Part model, mm, in its own coordinate system. A direction names the side the tool comes from. Round coordinates to 2 decimals unless told otherwise and drop trailing zeros. Loops run counter-clockwise (first coordinate to the right, second up) from the corner with the lowest first, then second, coordinate; pieces in that order, holes last. Notation, with made-up numbers: (-26, 82.5) - (15, 82.5) arc R27 cw to (15, 102.5) - close; hole circle Ø11 at (79.25, 16). An arc over 180 degrees is marked (long way). Write each question's results on one line, items separated by ' | '. Start each with the question number.
(1) Flat gauge pin, fed straight in: P1, Ø3.5, axis at x = 25.25, y = 20, coming from the -Z side. Where does the tip first touch, or does it go through?
(2) Cut at C-C, the plane x = 53.5. List the corners of the cut face in (y, z).
(3) Cut at D-D, the plane z = 1. Give the number of separate pieces and of enclosed holes in the cut face, then the cut area to 3 significant figures.
(4) Cut at A-A, the plane x = 6. List the corners of the cut face in (y, z).
(5) Mould opens along X. For faces 3 (the face through (10.6, -19.14, 0.99)), 4 (the face through (-12, 0, 0)), 5 (the face through (-76.64, 24.1, 1.01)) say: released by +X, released by -X, zero draft, split by the parting line, or undercut.
(6) Cut at B-B, the plane y = -8. List the corners of the cut face in (x, z).
(7) Tool access for faces 1 (the face through (29.15, 22.14, 0.99)), 2 (the face through (-76.64, -24.1, 1.01)): list every direction of +Z, -Z, +X, -X, +Y, -Y with a clear straight run to the whole face (end or side of a thin tool).
(8) Drill centre lines: L1, parallel to X at y = 10.5, z = 1.7; L2, parallel to X at y = 4.5, z = 1; L3, parallel to Y at x = -74.25, z = 1.4. Where is each one in solid material? Low to high.
from build123d import *

# Parameters (mm, degrees)
SKETCH_1_W          = 155
SKETCH_1_H          = 50
EXTRUDE_1_DEPTH     = 2
SKETCH_2_R          = 1.5
CUT_EXTRUDE_1_DEPTH = 10
FILLET_1_R          = 3
SKETCH_3_W          = 43
SKETCH_3_H          = 46
CUT_EXTRUDE_2_DEPTH = 10
FILLET_2_R          = 3
SKETCH_4_W          = 23
SKETCH_4_H          = 40
CUT_EXTRUDE_3_DEPTH = 10
FILLET_3_R          = 3
SKETCH_5_R          = 4.732430395
SKETCH_5_R_2        = 4.815282463
SKETCH_5_R_3        = 4.035251629
CUT_EXTRUDE_4_DEPTH = 10


with BuildPart() as part:
    # 草图1 → 凸台-拉伸1 (new body)
    with BuildSketch(Plane.XY):
        Rectangle(SKETCH_1_W, SKETCH_1_H)
    extrude(amount=EXTRUDE_1_DEPTH)

    # 草图2 → 切除-拉伸1 (cut)
    with BuildSketch(Plane(origin=(0, 0, 0), x_dir=(-1, 0, 0), z_dir=(0, 0, -1))):
        with Locations((-25.25, -20)):
            Circle(SKETCH_2_R)
        with Locations((-74.25, -20)):
            Circle(SKETCH_2_R)
        with Locations((-25.25, 20)):
            Circle(SKETCH_2_R)
        with Locations((-74.25, 20)):
            Circle(SKETCH_2_R)
        with Locations((25.25, -20)):
            Circle(SKETCH_2_R)
        with Locations((74.25, -20)):
            Circle(SKETCH_2_R)
        with Locations((25.25, 20)):
            Circle(SKETCH_2_R)
        with Locations((74.25, 20)):
            Circle(SKETCH_2_R)
        with Locations((16, 2.5)):
            Circle(SKETCH_2_R)
        with Locations((16, 17.5)):
            Circle(SKETCH_2_R)
        with Locations((-16, 2.5)):
            Circle(SKETCH_2_R)
        with Locations((-16, 17.5)):
            Circle(SKETCH_2_R)
    extrude(amount=-CUT_EXTRUDE_1_DEPTH, mode=Mode.SUBTRACT)

    # 圆角1
    fillet_1_edges = [part.edges().sort_by_distance(p)[0] for p in [
        (77.5, -25, 1),
        (-77.5, -25, 1),
        (-77.5, 25, 1),
        (77.5, 25, 1),
    ]]
    fillet(fillet_1_edges, radius=FILLET_1_R)

    # 草图3 → 切除-拉伸2 (cut)
    with BuildSketch(Plane.XY.offset(2)):
        with Locations((49.75, 0)):
            Rectangle(SKETCH_3_W, SKETCH_3_H)
        with Locations((-49.75, 0)):
            Rectangle(SKETCH_3_W, SKETCH_3_H)
    extrude(amount=-CUT_EXTRUDE_2_DEPTH, mode=Mode.SUBTRACT)

    # 圆角2
    fillet_2_edges = [part.edges().sort_by_distance(p)[0] for p in [
        (71.25, 23, 1),
        (71.25, -23, 1),
        (28.25, -23, 1),
        (28.25, 23, 1),
        (-28.25, 23, 1),
        (-28.25, -23, 1),
        (-71.25, -23, 1),
        (-71.25, 23, 1),
    ]]
    fillet(fillet_2_edges, radius=FILLET_2_R)

    # 草图4 → 切除-拉伸3 (cut)
    with BuildSketch(Plane.XY.offset(2)):
        Rectangle(SKETCH_4_W, SKETCH_4_H)
    extrude(amount=-CUT_EXTRUDE_3_DEPTH, mode=Mode.SUBTRACT)

    # 圆角3
    fillet_3_edges = [part.edges().sort_by_distance(p)[0] for p in [
        (11.5, 20, 1),
        (11.5, -20, 1),
        (-11.5, -20, 1),
        (-11.5, 20, 1),
    ]]
    fillet(fillet_3_edges, radius=FILLET_3_R)

    # 草图5 → 切除-拉伸4 (cut)
    with BuildSketch(Plane.XY.offset(2)):
        with Locations((19.907240007, 10.387913302)):
            Circle(SKETCH_5_R)
        with Locations((18.386877163, -5.018430181)):
            Circle(SKETCH_5_R_2)
        with Locations((16.663799274, -17.890835592)):
            Circle(SKETCH_5_R_3)
        with Locations(Location((-16.663799274, -17.890835592, 0), (0, 0, 180))):
            Circle(SKETCH_5_R_3)
        with Locations(Location((-18.386877163, -5.018430181, 0), (0, 0, 180))):
            Circle(SKETCH_5_R_2)
        with Locations(Location((-19.907240007, 10.387913302, 0), (0, 0, 180))):
            Circle(SKETCH_5_R)
    extrude(amount=-CUT_EXTRUDE_4_DEPTH, mode=Mode.SUBTRACT)


solid = part.part
A:
1) P1: z = 0
2) outline: (-25, 0) - (-23, 0) - (-23, 2) - (-25, 2) - close; (23, 0) - (25, 0) - (25, 2) - (23, 2) - close
3) separate pieces: 1 | enclosed holes: 21 | area: 2,420 mm2
4) outline: (-25, 0) - (-20, 0) - (-20, 2) - (-25, 2) - close; (20, 0) - (25, 0) - (25, 2) - (20, 2) - close
5) face 3: undercut | face 4: zero draft | face 5: released by -X
6) outline: (-77.5, 0) - (-71.25, 0) - (-71.25, 2) - (-77.5, 2) - close; (-28.25, 0) - (-22.17, 0) - (-22.17, 2) - (-28.25, 2) - close; (-14.61, 0) - (-11.5, 0) - (-11.5, 2) - (-14.61, 2) - close; (11.5, 0) - (14.61, 0) - (14.61, 2) - (11.5, 2) - close; (22.17, 0) - (28.25, 0) - (28.25, 2) - (22.17, 2) - close; (71.25, 0) - (77.5, 0) - (77.5, 2) - (71.25, 2) - close
7) face 1: +Z, -Z | face 2: +Z, -Z, -X, -Y
8) L1: -77.5 to -71.25, -28.25 to -24.64, -15.18 to -11.5, 11.5 to 15.18, 24.64 to 28.25, 71.25 to 77.5 | L2: -77.5 to -71.25, -28.25 to -11.5, 11.5 to 28.25, 71.25 to 77.5 | L3: -25 to -21.5, -18.5 to 18.5, 21.5 to 25
